Build history of the part. All positions in model axes, mm. A direction names the side the tool comes from. Round coordinates to 2 decimals unless told otherwise and drop trailing zeros. Write each loop counter-clockwise with the first axis right and the second up, starting at its lowest first coordinate (ties: lowest second). Pieces come first, ordered by that corner, then holes.
Item 1: Drop flat-ended pins along their axis: pin 1 Ø1.3 at (x, y) = (120.5, -1) entering from +Z; pin 2 Ø1.8 at (x, y) = (182, -0.5) entering from +Z; pin 3 Ø1.5 at (y, z) = (5.375, -5.625) entering from +X; pin 4 Ø2.5 at (y, z) = (-0.5, 1.5) entering from +X. Give the stop position or say it passes through.
Item 2: 3-axis set-ups, long thin cutter, end or side, ignore diameter. For faces 1 (the flat face through (311, 0, 0)), 2 (the flat face through (154, 0, -8)), 3 (the flat face through (2, 0, 0)), 4 (the flat face through (1.65, 5, -7)), 5 (the flat face through (156, -1, -11.25)): which of +Z, -Z, +X, -X, +Y, -Y reach the whole face in a straight line?
Item 3: Mould opens along X. For faces 6 (the flat face through (312.663, 5, -4)), 7 (the flat face through (311.013, 5, -4)), 8 (the flat face through (0, 5, -7)), 9 (the flat face through (154, -1.65, -8)) say: +X half, -X half, draft (parallel to the pull), parting line (faces both ways), or undercut.
Item 4: Band-saw the part on A-A, the plane x = 207. Write the cut outline in (y, z) (3 decimals), then the cut area to 3 significant figures.
Item 5: Wall check: probe 1 along Z at (x, y) = (76.5, -1); probe 2 along X at (y, z) = (4, -7.25); probe 3 along Y at (x, z) = (154.5, -8). Give the ranges that are in metal, low to high.
```python
from build123d import *

# Parameters (mm, degrees)
SKETCH1_W                             = 312.6632
SKETCH1_H                             = 11.25
BASE_FLANGE1_DEPTH                    = 1.65
EDGE_FLANGE1_STRIP_W                  = 9.9
EDGE_FLANGE1_STRIP_H                  = 1.65
EDGE_FLANGE1_STRIP_CUT_DEPTH          = 11.25
EDGE_FLANGE1_STRIP_2_W                = 9.9
EDGE_FLANGE1_STRIP_2_H                = 1.65
EDGE_FLANGE1_STRIP_CUT_2_DEPTH        = 11.25
EDGE_FLANGE1_DEPTH                    = 11.25
EDGE_FLANGE1_BEND_DEPTH               = 11.25
TAP_DRILL_FOR_M3X0_5_TAP1_D           = 2.5
TAP_DRILL_FOR_M3X0_5_TAP1_ON_FACE_2_D = 2.5
FILLET1_R                             = 2
CUT_EXTRUDE1_REACH                    = 314.988
EDGE_FLANGE2_DEPTH                    = 296.0632
FILLET2_R                             = 3


# Sheet-metal steps are written as plain solids
with BuildPart() as part:
    # Sketch1 → Base-Flange1 (new body)
    with BuildSketch(Plane(origin=(0, 0, 0), x_dir=(1, 0, 0), z_dir=(0, 1, 0))):
        with Locations((156.3316, 5.625)):
            Rectangle(SKETCH1_W, SKETCH1_H)
    extrude(amount=-BASE_FLANGE1_DEPTH)

    # Edge-Flange1 strip (across the edge) → Edge-Flange1 strip cut (cut)
    with BuildSketch(Plane.XY.offset(-11.25)):
        with Locations((-1.65, -0.825)):
            Rectangle(EDGE_FLANGE1_STRIP_W, EDGE_FLANGE1_STRIP_H)
    extrude(amount=EDGE_FLANGE1_STRIP_CUT_DEPTH, mode=Mode.SUBTRACT)

    # Edge-Flange1 strip 2 (across the edge) → Edge-Flange1 strip cut 2 (cut)
    with BuildSketch(Plane(origin=(312.6632, 0, 0), x_dir=(-1, 0, 0), z_dir=(0, 0, -1))):
        with Locations((-1.65, -0.825)):
            Rectangle(EDGE_FLANGE1_STRIP_2_W, EDGE_FLANGE1_STRIP_2_H)
    extrude(amount=EDGE_FLANGE1_STRIP_CUT_2_DEPTH, mode=Mode.SUBTRACT)

    # Edge-Flange1 section (across the edge) → Edge-Flange1 (add)
    with BuildSketch(Plane.XY.offset(-11.25)):
        with BuildLine():
            Line((0, 1.65), (0, 8.75))
            Line((0, 8.75), (1.65, 8.75))
            Line((1.65, 8.75), (1.65, 1.65))
            ThreePointArc((1.65, 1.65), (2.133273811, 0.483273811), (3.3, 0))
            Line((3.3, 0), (3.3, -1.65))
            ThreePointArc((3.3, -1.65), (0.966547622, -0.683452378), (0, 1.65))
        make_face()
    extrude(amount=EDGE_FLANGE1_DEPTH)

    # Edge-Flange1 section 2 (across the edge) → Edge-Flange1 bend (add)
    with BuildSketch(Plane(origin=(312.6632, 0, 0), x_dir=(-1, 0, 0), z_dir=(0, 0, -1))):
        with BuildLine():
            Line((0, 1.65), (0, 8.75))
            Line((0, 8.75), (1.65, 8.75))
            Line((1.65, 8.75), (1.65, 1.65))
            ThreePointArc((1.65, 1.65), (2.133273811, 0.483273811), (3.3, 0))
            Line((3.3, 0), (3.3, -1.65))
            ThreePointArc((3.3, -1.65), (0.966547622, -0.683452378), (0, 1.65))
        make_face()
    extrude(amount=EDGE_FLANGE1_BEND_DEPTH)

    # Tap Drill for M3x0.5 Tap1 (through all)
    with Locations(Plane(origin=(312.6632, 5.375, -5.625), x_dir=(0, 1, 0), z_dir=(1, 0, 0))):
        with Locations((0, 0)):
            Hole(TAP_DRILL_FOR_M3X0_5_TAP1_D / 2)

    # Tap Drill for M3x0.5 Tap1 on face 2 (through all)
    with Locations(Plane(origin=(0, 5.375, -5.625), x_dir=(0, 0, -1), z_dir=(-1, 0, 0))):
        with Locations((0, 0)):
            Hole(TAP_DRILL_FOR_M3X0_5_TAP1_ON_FACE_2_D / 2)

    # Fillet1
    fillet1_edges = [part.edges().sort_by_distance(p)[0] for p in [
        (0.825, 8.75, -11.25),
        (0.825, 8.75, 0),
        (311.8382, 8.75, 0),
        (311.8382, 8.75, -11.25),
    ]]
    fillet(fillet1_edges, radius=FILLET1_R)

    # Sketch15 → Cut-Extrude1 (cut, up to next)
    with BuildSketch(Plane(origin=(0, 0, 0), x_dir=(1, 0, 0), z_dir=(0, 1, 0)), mode=Mode.PRIVATE) as cut_extrude1_sk1:
        with BuildLine():
            Line((11.8, 8.125), (76.3, 8.125))
            ThreePointArc((76.3, 8.125), (78.8, 5.625), (76.3, 3.125))
            Line((76.3, 3.125), (11.8, 3.125))
            ThreePointArc((11.8, 3.125), (9.3, 5.625), (11.8, 8.125))
        make_face()
    cut_extrude1_tool1 = extrude(cut_extrude1_sk1.sketch, amount=-CUT_EXTRUDE1_REACH, mode=Mode.PRIVATE) & part.part
    # Sketch15 → Cut-Extrude1 (cut, up to next)
    with BuildSketch(Plane(origin=(0, 0, 0), x_dir=(1, 0, 0), z_dir=(0, 1, 0)), mode=Mode.PRIVATE) as cut_extrude1_sk2:
        with BuildLine():
            Line((87.49, 8.125), (151.99, 8.125))
            ThreePointArc((151.99, 8.125), (154.49, 5.625), (151.99, 3.125))
            Line((151.99, 3.125), (87.49, 3.125))
            ThreePointArc((87.49, 3.125), (84.99, 5.625), (87.49, 8.125))
        make_face()
    cut_extrude1_tool2 = extrude(cut_extrude1_sk2.sketch, amount=-CUT_EXTRUDE1_REACH, mode=Mode.PRIVATE) & part.part
    # Sketch15 → Cut-Extrude1 (cut, up to next)
    with BuildSketch(Plane(origin=(0, 0, 0), x_dir=(1, 0, 0), z_dir=(0, 1, 0)), mode=Mode.PRIVATE) as cut_extrude1_sk3:
        with BuildLine():
            Line((163.18, 8.125), (227.68, 8.125))
            ThreePointArc((227.68, 8.125), (230.18, 5.625), (227.68, 3.125))
            Line((227.68, 3.125), (163.18, 3.125))
            ThreePointArc((163.18, 3.125), (160.68, 5.625), (163.18, 8.125))
        make_face()
    cut_extrude1_tool3 = extrude(cut_extrude1_sk3.sketch, amount=-CUT_EXTRUDE1_REACH, mode=Mode.PRIVATE) & part.part
    # Sketch15 → Cut-Extrude1 (cut, up to next)
    with BuildSketch(Plane(origin=(0, 0, 0), x_dir=(1, 0, 0), z_dir=(0, 1, 0)), mode=Mode.PRIVATE) as cut_extrude1_sk4:
        with BuildLine():
            Line((238.87, 8.125), (303.37, 8.125))
            ThreePointArc((303.37, 8.125), (305.87, 5.625), (303.37, 3.125))
            Line((303.37, 3.125), (238.87, 3.125))
            ThreePointArc((238.87, 3.125), (236.37, 5.625), (238.87, 8.125))
        make_face()
    cut_extrude1_tool4 = extrude(cut_extrude1_sk4.sketch, amount=-CUT_EXTRUDE1_REACH, mode=Mode.PRIVATE) & part.part
    add(cut_extrude1_tool1.solids().sort_by_distance((44.05, 0, -5.625))[0], mode=Mode.SUBTRACT)
    add(cut_extrude1_tool2.solids().sort_by_distance((119.74, 0, -5.625))[0], mode=Mode.SUBTRACT)
    add(cut_extrude1_tool3.solids().sort_by_distance((195.43, 0, -5.625))[0], mode=Mode.SUBTRACT)
    add(cut_extrude1_tool4.solids().sort_by_distance((271.12, 0, -5.625))[0], mode=Mode.SUBTRACT)

    # Edge-Flange2 section (across the edge) → Edge-Flange2 (add)
    with BuildSketch(Plane(origin=(8.3, 0, 1.65), x_dir=(0, 0, -1), z_dir=(1, 0, 0))):
        with BuildLine():
            Line((-1.65, 1.65), (-1.65, 5))
            Line((-1.65, 5), (0, 5))
            Line((0, 5), (0, 1.65))
            ThreePointArc((0, 1.65), (0.483273811, 0.483273811), (1.65, 0))
            Line((1.65, 0), (1.65, -1.65))
            ThreePointArc((1.65, -1.65), (-0.683452378, -0.683452378), (-1.65, 1.65))
        make_face()
    extrude(amount=EDGE_FLANGE2_DEPTH)

    # Fillet2
    fillet2_edges = [part.edges().sort_by_distance(p)[0] for p in [
        (8.3, 5, 2.475),
        (304.3632, 5, 2.475),
    ]]
    fillet(fillet2_edges, radius=FILLET2_R)


solid = part.part
```
Results:
1. pin 1: stops at z = 2.62
1. pin 2: stops at z = 3.05
1. pin 3: passes through
1. pin 4: stops at x = 304.36
2. face 1: +Z, +X, +Y, -Y
2. face 2: -Z, +Y
2. face 3: +Z, -X, +Y, -Y
2. face 4: +Z, -Z, +Y
2. face 5: -Z, +X, -X, +Y, -Y
3. face 6: +X half
3. face 7: undercut
3. face 8: -X half
3. face 9: draft
4. outline: (-1.65, -11.25) - (0, -11.25) - (0, -8.125) - (-1.65, -8.125) - close; (-1.65, -3.125) - (0, -3.125) - (0, 0) arc R1.65 cw to (1.65, 1.65) - (5, 1.65) - (5, 3.3) - (1.65, 3.3) arc R3.3 ccw to (-1.65, 0) - close
4. area: 22.3 mm2
5. probe 1: z = -11.25 to -8.12, -3.13 to 1.97
5. probe 2: x = 0 to 1.65, 311.01 to 312.66
5. probe 3: y = -1.65 to 0
